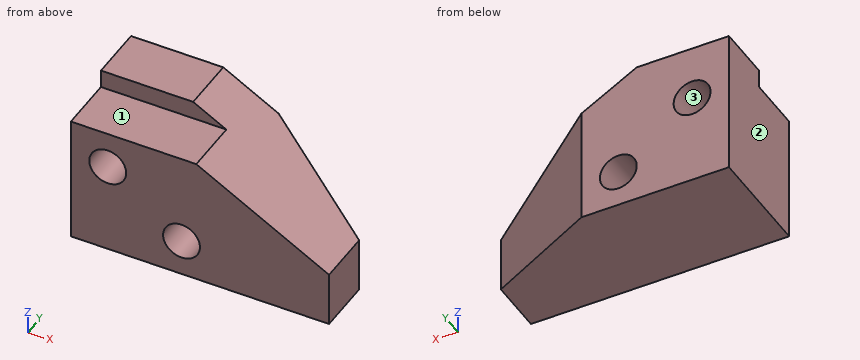
```python
from build123d import *

# Parameters (mm, degrees)
SKETCH1_W           = 70
SKETCH1_H           = 40
BOSS_EXTRUDE1_DEPTH = 30
CUT_EXTRUDE1_DEPTH  = 41
CUT_EXTRUDE2_DEPTH  = 31
SKETCH5_W           = 5
SKETCH5_H           = 15
CUT_EXTRUDE3_DEPTH  = 71
SKETCH6_R           = 5
CUT_EXTRUDE4_DEPTH  = 31
SKETCH7_R           = 5
CUT_EXTRUDE5_DEPTH  = 31


with BuildPart() as part:
    # Sketch1 → Boss-Extrude1 (new body)
    with BuildSketch(Plane(origin=(0, 0, 0), x_dir=(1, 0, 0), z_dir=(0, 1, 0))):
        with Locations((35, 20)):
            Rectangle(SKETCH1_W, SKETCH1_H)
    extrude(amount=BOSS_EXTRUDE1_DEPTH)

    # Sketch2 → Cut-Extrude1 (cut, through all)
    with BuildSketch(Plane.XY):
        Polygon((70, 30), (40, 30), (70, 15), align=None)
    extrude(amount=-CUT_EXTRUDE1_DEPTH, mode=Mode.SUBTRACT)

    # Sketch4 → Cut-Extrude2 (cut, through all)
    with BuildSketch(Plane(origin=(0, 0, 0), x_dir=(-1, 0, 0), z_dir=(0, -1, 0))):
        Polygon((-25, 0), (-70, 25), (-70, 0), align=None)
    extrude(amount=-CUT_EXTRUDE2_DEPTH, mode=Mode.SUBTRACT)

    # Sketch5 → Cut-Extrude3 (cut, through all)
    with BuildSketch(Plane.ZY):
        with Locations((-2.5, 7.5)):
            Rectangle(SKETCH5_W, SKETCH5_H)
    extrude(amount=-CUT_EXTRUDE3_DEPTH, mode=Mode.SUBTRACT)

    # Sketch6 → Cut-Extrude4 (cut, through all)
    with BuildSketch(Plane(origin=(0, 30, 0), x_dir=(1, 0, 0), z_dir=(0, 1, 0))):
        with Locations((10, 15)):
            Circle(SKETCH6_R)
    extrude(amount=-CUT_EXTRUDE4_DEPTH, mode=Mode.SUBTRACT)

    # Sketch7 → Cut-Extrude5 (cut, through all)
    with BuildSketch(Plane(origin=(0, 30, 0), x_dir=(1, 0, 0), z_dir=(0, 1, 0))):
        with Locations((30, 30)):
            Circle(SKETCH7_R)
    extrude(amount=-CUT_EXTRUDE5_DEPTH, mode=Mode.SUBTRACT)


solid = part.part
```
Verification items for the finished model (mm, model axes). Face numbers are marked on the shaded views. Give positions to 0.01 mm unless a question says otherwise; leave off trailing zeros. Order: outer loops, then holes, each group sorted by start corner. A loop starts at its lowest first (then second) coordinate and runs counter-clockwise, first axis right, second up. Notation, with made-up numbers: (-27.75, -39) - (-11.75, -39) arc R14 cw to (-11.75, -12) - close; hole circle Ø1 at (-17.75, 46). An arc over 180 degrees is marked (long way). Answer as CSV lines item,"result". Start each with the question number.
Item 1: Section check B-B, the plane x = 10. Record the boundary of the cut face in (y, z).
Item 2: Gauge pin test, flat ends, axial feed: pin 1 (12 mm diameter, centred on x = 15.5, y = 8.5, fed in from +Z); pin 2 (12 mm diameter, centred on x = 10, z = -35.5, fed in from -Y); pin 3 (2.5 mm diameter, centred on x = 17.5, z = -3, fed in from -Y); pin 4 (5 mm diameter, centred on y = 15, z = -9, fed in from +X). Record the tip position at first contact, or that the pin passes through.
Item 3: Mould release check, pull along Z, two halves, no side actions. Record for the marked faces 1, 2 and 3: released by +Z, released by -Z, zero draft, split by the parting line, or undercut.
Item 4: Material ranges on L1, parallel to X at y = 12.75, z = -30; L2, parallel to Z at x = 10, y = 23.25; L3, parallel to Z at x = 30, y = 9, recorded low to high.
Item 5: Section check A-A, the plane z = -30. Record the boundary of the cut face in (x, y), plus the area to 4 significant figures.
Item 6: Section check C-C, the plane y = 13. Record the boundary of the cut face in (x, z).
Item 7: Section check D-D, the plane z = -22. Record the boundary of the cut face in (x, y).
Filled in:
1,outline,"(0, -40) - (30, -40) - (30, -20) - (0, -20) - close; (0, -10) - (30, -10) - (30, 0) - (15, 0) - (15, -5) - (0, -5) - close"
2,pin 1,"z = -5"
2,pin 2,"y = 0"
2,pin 3,"y = 15"
2,pin 4,"x = 45.7"
3,face 1,"released by +Z"
3,face 2,"zero draft"
3,face 3,"undercut"
4,L1,"0 to 25, 35 to 70"
4,L2,"-40 to -20, -10 to 0"
4,L3,"-40 to -35, -25 to -5"
5,outline,"(0, 0) - (25, 0) - (25, 30) - (0, 30) - close; (35, 0) - (70, 0) - (70, 15) - (40, 30) - (35, 30) - close"
5,area,"1,575 mm^2"
6,outline,"(0, -40) - (70, -40) - (70, -25) - (34, -5) - (0, -5) - close; hole circle Ø10 at (10, -15); hole circle Ø10 at (30, -30)"
7,outline,"(0, 0) - (64.6, 0) - (64.6, 17.7) - (40, 30) - (0, 30) - close"
